Check sheet for the modelled part. Datum: model origin and axes. Units: mm. Round coordinates to 2 decimals unless told otherwise and drop trailing zeros. Write each loop counter-clockwise with the first axis right and the second up, starting at its lowest first coordinate (ties: lowest second). Pieces come first, ordered by that corner, then holes.
from build123d import *

# Parameters (mm, degrees)
SKETCH1_R                = 45
BOSS_EXTRUDE1_DEPTH      = 2
F_8_0MM_DOWEL_HOLE1_D    = 15
F_3_0_3_DIAMETER_HOLE1_D = 3


with BuildPart() as part:
    # Sketch1 → Boss-Extrude1 (new body)
    with BuildSketch(Plane(origin=(0, 0, 0), x_dir=(1, 0, 0), z_dir=(0, 1, 0))):
        with Locations(Location((0, 0, 0), (0, 0, 270))):
            Circle(SKETCH1_R)
    extrude(amount=-BOSS_EXTRUDE1_DEPTH)

    # Ø8.0mm Dowel Hole1 (through all)
    with Locations(Plane(origin=(0, 0, 0), x_dir=(1, 0, 0), z_dir=(0, 1, 0))):
        with Locations((-16.606971943, 28.764119165), (-16.606971943, -28.764119165), (33.213943886, 0), (16.606971943, 28.764119165), (16.606971943, -28.764119165), (-33.213943886, 0)):
            Hole(F_8_0MM_DOWEL_HOLE1_D / 2)

    # Ø3.0 (3) Diameter Hole1 (through all)
    with Locations(Plane(origin=(0, 0, 0), x_dir=(1, 0, 0), z_dir=(0, 1, 0))):
        with Locations((-34.641016151, 20), (0, -40), (34.641016151, 20)):
            Hole(F_3_0_3_DIAMETER_HOLE1_D / 2)


solid = part.part
1. Scan lines: line 1 along X through (y, z) = (-0.3, -0.5); line 2 along Z through (x, y) = (-21, -0.4); line 3 along X through (y, z) = (-1.2, -20). Record each from-to range of solid material in increasing order.
2. Sectioned sample at A-A, the plane z = 0. Enter the section's corners in (x, y).
3. Release check for a two-part mould opening along X. For faces 1 (the cylindrical face through (-17.235, -0.986, 41.569)), 2 (the cylindrical face through (-34.446, -1.014, -21.487)), 3 (the flat face through (1, 0, -1)) record: released by +X, released by -X, zero draft, split by the parting line, or undercut.
4. Sectioned sample at C-C, the plane x = -13.5. Enter the section's corners in (y, z), plus the area to 3 significant figures.
5. Sectioned sample at B-B, the plane x = 0. Enter the section's corners in (y, z).
6. Sectioned sample at D-D, the plane z = 40. Enter the section's corners in (x, y).
7. Go/stop test with flat-tipped pins: pin 1 (13.5 mm diameter, centred on x = -16.61, z = -28.76, fed in from +Y); pin 2 (1 mm diameter, centred on y = -1.5, z = -13.5, fed in from -X). Record where each tip stops, or that it passes through.
Computed values:
1. line 1: x = -45 to -40.7, -25.73 to 25.73, 40.7 to 45
1. line 2: z = -39.8 to -34.84, -22.69 to 22.69, 34.84 to 39.8
1. line 3: x = -40.31 to -36.14, -33.14 to 33.14, 36.14 to 40.31
2. outline: (-45, -2) - (-40.71, -2) - (-40.71, 0) - (-45, 0) - close; (-25.71, -2) - (25.71, -2) - (25.71, 0) - (-25.71, 0) - close; (40.71, -2) - (45, -2) - (45, 0) - (40.71, 0) - close
3. face 1: split by the parting line
3. face 2: undercut
3. face 3: zero draft
4. outline: (-2, -42.93) - (0, -42.93) - (0, -35.59) - (-2, -35.59) - close; (-2, -21.94) - (0, -21.94) - (0, 21.94) - (-2, 21.94) - close; (-2, 35.59) - (0, 35.59) - (0, 42.93) - (-2, 42.93) - close
4. area: 117 mm2
5. outline: (-2, -45) - (0, -45) - (0, 38.5) - (-2, 38.5) - close; (-2, 41.5) - (0, 41.5) - (0, 45) - (-2, 45) - close
6. outline: (-20.62, -2) - (-1.5, -2) - (-1.5, 0) - (-20.62, 0) - close; (1.5, -2) - (20.62, -2) - (20.62, 0) - (1.5, 0) - close
7. pin 1: passes through
7. pin 2: stops at x = -43.08
